Can you work these out from the model? Positions are in its coordinate system, mm. A direction names the side the tool comes from. Coordinates: 2 decimals unless noted, no trailing zeros. Order: outer loops, then holes, each group sorted by start corner. A loop starts at its lowest first (then second) coordinate and runs counter-clockwise, first axis right, second up. Notation, with made-up numbers: (87.25, -25) -> (141.25, -25) arc R37 ccw to (141.25, 13) -> close; hole circle Ø4 at (80.25, 12). An arc over 180 degrees is marked (long way). Write item = value, one per line.
Autodesk Inventor part; units mm, degrees
ref_plane "YZ Plane" through (0, 0, 0) normal (1, 0, 0) x (0, 1, 0)
ref_plane "XZ Plane" through (0, 0, 0) normal (0, 1, 0) x (-1, 0, 0)
ref_plane "XY Plane" through (0, 0, 0) normal (0, 0, 1) x (1, 0, 0)
sketch "Esquisse1" plane through (0, 0, 0) normal (0, 0, 1) x (1, 0, 0)
  point P0 (0, 0)
sketch "Esquisse2" plane through (0, 0, 0) normal (0, 0, 1) x (1, 0, 0)
  line L0 (0, 0) -> (20, 0)
  line L1 (20, 0) -> (20, 100)
  line L2 (20, 100) -> (0, 100)
  line L3 (0, 100) -> (0, 0)
  dimension "d0" = 100
  dimension "d1" = 20
extrude "Extrusion1" add sketch "Esquisse2" along normal blind 5
sketch "Esquisse3" plane through (0, 0, 5) normal (0, 0, 1) x (1, 0, 0)
  line L0 (20, 100) -> (0, 100)
  line L1 (0, 0) -> (20, 0)
  line L2 (7.5, 100) -> (12.5, 100)
  line L3 (12.5, 100) -> (12.5, 0)
  line L4 (12.5, 0) -> (7.5, 0)
  line L5 (7.5, 0) -> (7.5, 100)
  line L6 (20, 0) -> (20, 100)
  line L7 (0, 100) -> (0, 0)
  dimension "d4" = 7.5
  dimension "d5" = 7.5
extrude "Extrusion2" add sketch "Esquisse3" along normal blind 7.5 and the other way blind 12.5 contours L3 L1 L5 L0
sketch "Esquisse4" plane through (0, 0, 12.5) normal (0, 0, 1) x (1, 0, 0)
  line L0 (12.5, 0) -> (12.5, 100)
  line L1 (7.5, 0) -> (12.5, 0)
  line L2 (12.5, 0) -> (12.5, 15)
  line L3 (12.5, 15) -> (7.5, 15)
  line L4 (7.5, 15) -> (7.5, 0)
  point P0 (0, 0)
  dimension "d10" = 15
extrude "Extrusion3" add sketch "Esquisse4" along normal blind 30 and the other way blind 50
sketch "Esquisse5" plane through (0, 0, 0) normal (-1, 0, 0) x (0, 0, 1)
  line L0 (5, 100) -> (5, 0)
  line L1 (0, 0) -> (5, 0)
  line L2 (5, 0) -> (5, 15)
  line L3 (5, 15) -> (0, 15)
  line L4 (0, 15) -> (0, 0)
  dimension "d15" = 15
extrude "Extrusion4" add sketch "Esquisse5" along normal blind 30 and the other way blind 50
sketch "Esquisse6" plane through (0, 100, 0) normal (-1, 0, 0) x (0, 0, 1)
  line L0 (5, 0) -> (5, -85)
  line L1 (0, -50) -> (5, -50)
  line L2 (5, -50) -> (5, -40)
  line L3 (5, -40) -> (0, -40)
  line L4 (0, -40) -> (0, -50)
  line L5 (0, 0) -> (5, 0)
  line L6 (0, -85) -> (5, -85)
  point P0 (0, -100)
  dimension "d20" = 40
  dimension "d22" = 35
extrude "Extrusion5" add sketch "Esquisse6" along normal blind 30 and the other way blind 50
sketch "Esquisse7" plane through (20, 60, 5) normal (0, 1, 0) x (1, 0, 0)
  line L0 (-20, 5) -> (-50, 5)
  line L1 (-50, 0) -> (-45, 0)
  line L2 (-45, 0) -> (-45, 5)
  line L3 (-45, 5) -> (-50, 5)
  line L4 (-50, 5) -> (-50, 0)
  dimension "d27" = 5
  dimension "d28" = 5
  dimension "d29" = 5
extrude "Extrusion6" add sketch "Esquisse7" along normal blind 10 and the other way blind 20
sketch "Esquisse8" plane through (20, 60, 5) normal (0, 1, 0) x (1, 0, 0)
  line L0 (30, 0) -> (25, 0)
  line L1 (25, 0) -> (25, 5)
  line L2 (25, 5) -> (30, 5)
  line L3 (30, 5) -> (30, 0)
  point P0 (-20, 5)
  dimension "d34" = 5
  dimension "d35" = 5
extrude "Extrusion7" add sketch "Esquisse8" along normal blind 10 and the other way blind 20
sketch "Esquisse9" plane through (0, 0, -7.5) normal (0, 0, -1) x (-1, 0, 0)
  line L0 (-7.5, 15) -> (-7.5, 100)
  line L1 (-12.5, 60) -> (-7.5, 60)
  line L2 (-7.5, 60) -> (-7.5, 50)
  line L3 (-7.5, 50) -> (-12.5, 50)
  line L4 (-12.5, 50) -> (-12.5, 60)
  line L5 (-7.5, 100) -> (-12.5, 100)
  line L6 (-12.5, 15) -> (-7.5, 15)
  point P0 (0, 0)
  dimension "d40" = 5
  dimension "d41" = 40
  dimension "d42" = 35
extrude "Extrusion8" add sketch "Esquisse9" along normal blind 30 and the other way blind 50
sketch "Esquisse10" plane through (7.5, 60, 12.5) normal (0, 1, 0) x (1, 0, 0)
  line L0 (0, 0) -> (0, -30)
  line L1 (5, -30) -> (0, -30)
  line L2 (0, -30) -> (0, -25)
  line L3 (0, -25) -> (5, -25)
  line L4 (5, -25) -> (5, -30)
  point P0 (-7.5, 12.5)
  dimension "d47" = 5
extrude "Extrusion9" add sketch "Esquisse10" along normal blind 10 and the other way blind 20
sketch "Esquisse11" plane through (7.5, 60, -7.5) normal (0, 1, 0) x (1, 0, 0)
  line L0 (5, 0) -> (5, 30)
  line L1 (0, 30) -> (5, 30)
  line L2 (5, 30) -> (5, 25)
  line L3 (5, 25) -> (0, 25)
  line L4 (0, 25) -> (0, 30)
  point P0 (-7.5, -7.5)
  dimension "d52" = 5
extrude "Extrusion10" add sketch "Esquisse11" along normal blind 10 and the other way blind 20
Item 1: I want a section at D-D, the plane y = 16.5. Please give me the cut outline in (x, z).
A:
outline = (0, 0) -> (7.5, 0) -> (7.5, -7.5) -> (12.5, -7.5) -> (12.5, 0) -> (20, 0) -> (20, 5) -> (12.5, 5) -> (12.5, 12.5) -> (7.5, 12.5) -> (7.5, 5) -> (0, 5) -> close
Item 2: For faces 1 (the flat face through (-28, 70, 2)), 2 (the flat face through (47, 40, 2)), 3 (the flat face through (12.5, 40, -7)), 4 (the flat face through (10, 50, -20)), 5 (the flat face through (45, 65, 3)), which set-ups out of +Z, -Z, +X, -X, +Y, -Y let a thin tool reach every point of the face, with its end or its side?
A:
face_1 = +Z, -Z, -X, +Y
face_2 = +Z, -Z, +X
face_3 = -Z, +X, +Y, -Y
face_4 = +X, -X
face_5 = +Z, -Z, +Y
Item 3: If I drill on probe 1 along Y at (x, z) = (10, 34); probe 2 along X at (y, z) = (49, 9); probe 3 along Z at (x, y) = (4, 69), over which ranges is the centre line in solid material (lowest first)?
A:
probe_1 = 0 to 15, 50 to 60
probe_2 = 7.5 to 12.5
probe_3 = 0 to 5
Item 4: I'm going to push flat-ended pins straight in: P1, Ø1.5, axis at y = 30, z = 3, coming from the -X side; P2, Ø12, axis at x = -18.5, y = 70.5, coming from the +Z side; P3, Ø10, axis at y = 43.5, z = -6, coming from the -X side; P4, Ø5.5, axis at x = -6.5, z = 1.5, coming from the +Y side. Where does each tip first touch, or does it pass through?
A:
P1 = 0
P2 = through
P3 = 7.5
P4 = 60
Item 5: I want a section at C-C, the plane x = -2. Please give me the cut outline in (y, z).
A:
outline = (0, 0) -> (15, 0) -> (15, 5) -> (0, 5) -> close; (50, 0) -> (60, 0) -> (60, 5) -> (50, 5) -> close
Item 6: I want a section at A-A, the plane z = 16.5. Please give me the cut outline in (x, y).
A:
outline = (7.5, 0) -> (12.5, 0) -> (12.5, 15) -> (7.5, 15) -> close; (7.5, 50) -> (12.5, 50) -> (12.5, 60) -> (7.5, 60) -> close
Item 7: I want a section at B-B, the plane y = 46. Please give me the cut outline in (x, z), plus the area to 3 significant figures.
A:
outline = (-30, 0) -> (-25, 0) -> (-25, 5) -> (-30, 5) -> close; (0, 0) -> (7.5, 0) -> (7.5, -7.5) -> (12.5, -7.5) -> (12.5, 0) -> (20, 0) -> (20, 5) -> (12.5, 5) -> (12.5, 12.5) -> (7.5, 12.5) -> (7.5, 5) -> (0, 5) -> close; (7.5, -37.5) -> (12.5, -37.5) -> (12.5, -32.5) -> (7.5, -32.5) -> close; (7.5, 37.5) -> (12.5, 37.5) -> (12.5, 42.5) -> (7.5, 42.5) -> close; (45, 0) -> (50, 0) -> (50, 5) -> (45, 5) -> close
area = 275 mm2
Item 8: If we mould it in two halves opening along X, with no side actions, what happens to faces 6 (the flat face through (50, 55, 2)), 7 (the flat face through (10, 70, -35)), 8 (the flat face through (-25, 65, 3)), 9 (the flat face through (20, 80, 2))? For each: pulls with the +X half, pulls with the -X half, needs draft (parallel to the pull), parting line crosses it, or undercut.
A:
face_6 = pulls with the +X half
face_7 = needs draft
face_8 = undercut
face_9 = undercut
